The model under review builds one solid part; all positions refer to its coordinate system, in mm. A direction names the side the tool comes from. Give positions to 0.01 mm unless a question says otherwise; leave off trailing zeros. Loops run counter-clockwise (first coordinate to the right, second up) from the corner with the lowest first, then second, coordinate; pieces in that order, holes last. Notation, with made-up numbers: M -15,-29 L -4,-29 A33 cw -4,-1 Z; hole C 17,66 d9. An arc over 180 degrees is marked long. Write item = value, one per line. Start each with the question number.
1. We need section D-D on z = 1.55. Count the separate pieces of the cut face and the enclosed holes in it, then the cut area to 3 significant figures.
2. Draft analysis for pull direction X (two halves, no side actions). For faces 1 (the face through (47.19, -1.94, 4)), 2 (the face through (42.38, 54.9, 0.18)), 3 (the face through (-42.5, 54.9, 3.2)), state which applies: pulls with the +X half, pulls with the -X half, needs draft (parallel to the pull), parting line crosses it, or undercut.
3. For pin 1 (8 mm diameter, centred on x = 46.25, y = 0, fed in from +Z), flat-tipped, find the tip position at first contact; note if it passes through.
4. For faces 4 (the face through (-49, 59.5, 3)), 5 (the face through (-52.5, 65, 3)), 6 (the face through (49, -59.5, 3)), 7 (the face through (50.542, 1.352, 4.507)), list the 3-axis set-ups (+Z, -Z, +X, -X, +Y, -Y) from which the entire face can be reached by the end or side of a thin tool; tool diameter is ignored.
5. Wall thickness on line 1 along Y through (x, z) = (0, 4.65); line 2 along Y through (x, z) = (-10, 4.8); line 3 along X through (y, z) = (36, 4.5): over which ranges is each line inside the solid? List them lowest first. Write a range as from..to.
6. We need section B-B on y = 65.25. Give the boundary of the cut face in (x, z), then the cut area to 3 significant figures.
Autodesk Inventor part; units mm, degrees
ref_plane "YZ Plane" through (0, 0, 0) normal (1, 0, 0) x (0, 1, 0)
ref_plane "XZ Plane" through (0, 0, 0) normal (0, 1, 0) x (-1, 0, 0)
ref_plane "XY Plane" through (0, 0, 0) normal (0, 0, 1) x (1, 0, 0)
sketch "Sketch1" plane through (0, 0, 0) normal (0, 0, 1) x (1, 0, 0)
  line L0 (-39.6, -58.6) -> (39.6, -58.6)
  line L1 (39.6, -58.6) -> (39.6, 58.6)
  line L2 (39.6, 58.6) -> (-39.6, 58.6)
  line L3 (-39.6, 58.6) -> (-39.6, -58.6)
  line L4 (-39.6, -58.6) -> (39.6, 58.6) construction
  line L5 (39.6, -58.6) -> (-39.6, 58.6) construction
  line L6 (-52.5, -71.5) -> (52.5, -71.5)
  line L7 (52.5, -71.5) -> (52.5, 71.5)
  line L8 (52.5, 71.5) -> (-52.5, 71.5)
  line L9 (-52.5, 71.5) -> (-52.5, -71.5)
  line L10 (-52.5, -71.5) -> (52.5, 71.5) construction
  line L11 (52.5, -71.5) -> (-52.5, 71.5) construction
  line L12 (0, 100.1) -> (0, -100.1)
  line L13 (-73.5, 0) -> (73.5, 0)
  circle A0 centre (-45.85, 0) radius 2
  circle A1 centre (46.25, 0) radius 2
  circle A2 centre (0, 65.25) radius 2
  circle A3 centre (0, -65.25) radius 2
  point P0 (0, 0)
  dimension "d0" = 79.2
  dimension "d1" = 117.2
  dimension "d2" = 105
  dimension "d4" = 12.9
  dimension "d6" = 6.25
  dimension "d7" = 6.25
  dimension "d8" = 6.25
  dimension "d9" = 6.25
  dimension "d10" = 4
  dimension "d11" = 4
  dimension "d12" = 4
  dimension "d40" = 143
  dimension "d41" = 4
extrude "Extrusion1" add sketch "Sketch1" along normal blind 6 contours L0 L12 A3 L6 L9 L13 A0 L3 | L0 L1 L13 A1 L7 L6 L12 A3 | L13 A0 L9 L8 L12 A2 L2 L3 | L1 L2 L12 A2 L8 L7 L13 A1
fillet "Fillet1" radius 2 8 edges at (-39.6, 58.6, 3) (39.6, 58.6, 3) (39.6, -58.6, 3) (-39.6, -58.6, 3) (52.5, 71.5, 3) (-52.5, 71.5, 3) (-52.5, -71.5, 3) (52.5, -71.5, 3)
sketch "Sketch2" plane through (0, 0, 6) normal (0, 0, 1) x (1, 0, 0)
  circle A0 centre (0, 65.25) radius 2
  circle A1 centre (46.25, 0) radius 2
  circle A2 centre (0, -65.25) radius 2
  circle A3 centre (-45.85, 0) radius 2
  circle A4 centre (0, 65.25) radius 4.5
  circle A5 centre (46.25, 0) radius 4.5
  circle A6 centre (0, -65.25) radius 4.5
  circle A7 centre (-45.85, 0) radius 4.5
  point P0 (0, 0)
  dimension "d16" = 9
  dimension "d17" = 9
  dimension "d18" = 9
  dimension "d19" = 9
extrude "Extrusion2" cut sketch "Sketch2" against normal blind 2
chamfer "Chamfer1" distance 1 angle 45 4 edges at (-4.5, 65.25, 6) (-50.35, 0, 6) (41.75, 0, 6) (-4.5, -65.25, 6)
sketch "Sketch3" plane through (0, 0, 6) normal (0, 0, 1) x (1, 0, 0)
  circle A0 centre (-47, -55) radius 4.5
  line L0 (-73.5, 0) -> (73.5, 0) construction
  line L1 (0, 100.1) -> (0, -100.1) construction
  line L2 (-47, -50.5) -> (-52.5, -50.5)
  line L3 (-52.5, 69.5) -> (-52.5, -69.5) construction
  line L4 (-52.5, -50.5) -> (-52.5, -59.5)
  line L5 (-52.5, -59.5) -> (-47, -59.5)
  circle A1 centre (47, -55) radius 4.5
  line L6 (47, -50.5) -> (52.5, -50.5)
  line L7 (52.5, -50.5) -> (52.5, -59.5)
  line L8 (52.5, -59.5) -> (47, -59.5)
  circle A2 centre (-47, 55) radius 4.5
  line L9 (-47, 50.5) -> (-52.5, 50.5)
  line L10 (-52.5, 50.5) -> (-52.5, 59.5)
  line L11 (-52.5, 59.5) -> (-47, 59.5)
  circle A3 centre (47, 55) radius 4.5
  line L12 (47, 50.5) -> (52.5, 50.5)
  line L13 (52.5, 50.5) -> (52.5, 59.5)
  line L14 (52.5, 59.5) -> (47, 59.5)
  point P0 (0, 0)
  dimension "d25" = 9
  dimension "d26" = 55
  dimension "d27" = 47
extrude "Extrusion3" cut sketch "Sketch3" against normal through all
chamfer "Chamfer2" distance 1 angle 45 8 edges at (-52.5, -50.5, 3) (-52.5, -59.5, 3) (52.5, -59.5, 3) (52.5, -50.5, 3) (52.5, 59.5, 3) (52.5, 50.5, 3) (-52.5, 59.5, 3) (-52.5, 50.5, 3)
sketch "Sketch4" plane through (0, 0, 0) normal (0, 0, -1) x (-1, 0, 0)
  line L0 (37.6, 58.6) -> (-37.6, 58.6)
  arc A0 (39.6, 56.6) -> (37.6, 58.6) centre (37.6, 56.6) ccw
  line L1 (39.6, -56.6) -> (39.6, 56.6)
  arc A1 (37.6, -58.6) -> (39.6, -56.6) centre (37.6, -56.6) ccw
  line L2 (-37.6, -58.6) -> (37.6, -58.6)
  arc A2 (-39.6, -56.6) -> (-37.6, -58.6) centre (-37.6, -56.6) ccw
  line L3 (-39.6, 56.6) -> (-39.6, -56.6)
  arc A3 (-37.6, 58.6) -> (-39.6, 56.6) centre (-37.6, 56.6) ccw
  line L4 (-37.6, 56.6) -> (37.6, 56.6)
  line L5 (37.6, 56.6) -> (37.6, -56.6)
  line L6 (37.6, -56.6) -> (-37.6, -56.6)
  line L7 (-37.6, -56.6) -> (-37.6, 56.6)
  point P0 (0, 0)
  point P1 (37.6, 56.6)
  point P2 (-37.6, -56.6)
  dimension "d33" = 2
extrude "Extrusion4" add sketch "Sketch4" against normal blind 0.5
fillet "Fillet2" radius 2 8 edges at (39.0142, 58.0142, 0.5) (39.6, 0, 0.5) (39.0142, -58.0142, 0.5) (0, -58.6, 0.5) (-39.0142, -58.0142, 0.5) (-39.6, 0, 0.5) (-39.0142, 58.0142, 0.5) (0, 58.6, 0.5)
chamfer "Chamfer3" distance 0.3 angle 45 28 edges at (0, 71.5, 0) (-51.9142, 70.9142, 0) (-52.5, 65, 0) (51.9142, 70.9142, 0) (52.5, 65, 0) (42.5, 55, 0) (49.25, 50.5, 0) (49.25, 59.5, 0) (52.5, 0, 0) (42.5, -55, 0) (49.25, -59.5, 0) (49.25, -50.5, 0) (52.5, -65, 0) (51.9142, -70.9142, 0) (0, -71.5, 0) (-51.9142, -70.9142, 0) (-52.5, -65, 0) (-42.5, -55, 0) (-49.25, -50.5, 0) (-49.25, -59.5, 0) (-52.5, 0, 0) (-49.25, 59.5, 0) (-42.5, 55, 0) (-49.25, 50.5, 0) (0, 56.6, 0) (-37.6, 0, 0) (37.6, 0, 0) (0, -56.6, 0)
equation "\"d7\" = d6"
equation "\"d8\" = d6"
equation "\"d9\" = d6"
equation "\"d11\" = d10"
equation "\"d12\" = d10"
equation "\"d41\" = d11"
equation "\"d17\" = d16"
equation "\"d18\" = d16"
equation "\"d19\" = d18"
properties part number "_3DPrint"
Final values:
q1.separate_pieces = 1
q1.enclosed_holes = 5
q1.area = 5,450 mm²
q2.face_1 = undercut
q2.face_2 = pulls with the +X half
q2.face_3 = pulls with the -X half
q3.pin_1 = 4
q4.face_4 = +Z, -Z, -X
q4.face_5 = +Z, -Z, -X, +Y, -Y
q4.face_6 = +Z, -Z, +X
q4.face_7 = +Z
q5.line_1 = -71.5..-69.75, -60.75..-58.6, 58.6..60.75, 69.75..71.5
q5.line_2 = -71.5..-58.6, 58.6..71.5
q5.line_3 = -52.5..-39.6, 39.6..52.5
q6.outline = M -52.5,0.3 L -52.2,0 L -2,0 L -2,4 L -4.5,4 L -4.5,5 L -5.5,6 L -52.5,6 Z; M 2,0 L 52.2,0 L 52.5,0.3 L 52.5,6 L 5.5,6 L 4.5,5 L 4.5,4 L 2,4 Z
q6.area = 595 mm²
